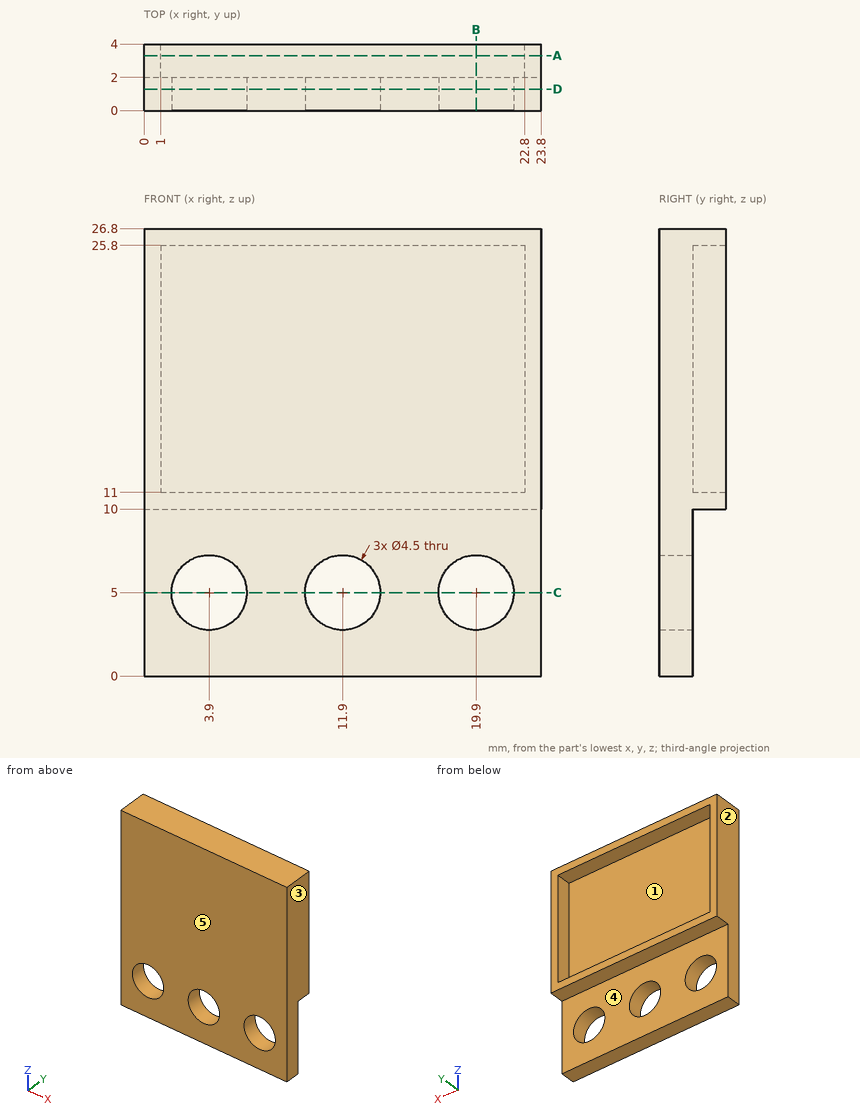
Job drawing, mm, ordinate dimensions from the low corner. One solid piece. A direction names the side the tool comes from. Coordinates: 2 decimals unless noted, no trailing zeros. Write each loop counter-clockwise with the first axis right and the second up, starting at its lowest first coordinate (ties: lowest second). Pieces come first, ordered by that corner, then holes.
Item 1: Slice it at A-A (y = 3.3). Write the cut outline in (x, z).
Item 2: Slice it at C-C (z = 5). Write the cut outline in (x, y).
Item 3: Pin check, flat tips, straight feed: pin 1 (6 mm diameter, centred on x = 19.9, z = 5, fed in from +Y); pin 2 (0.6 mm diameter, centred on x = 15.5, y = 2.5, fed in from -Z). Stop position of each tip, or through.
Item 4: Probe line 1 (X direction, y = 0.9, z = 5); line 2 (X direction, y = 2.7, z = 25.5); line 3 (Z direction, x = 7.25, y = 3.6). List the from-to ranges inside material, lowest first.
Item 5: Slice it at D-D (y = 1.3). Write the cut outline in (x, z), and give its area (3 significant figures).
Item 6: Which spindle directions (+Z, -Z, +X, -X, +Y, -Y) get a long thin tool onto all of the face, cutting with end or side? Do the marked faces 4 and 5. Say none if no direction does.
Item 7: Slice it at B-B (x = 19.9). Write the cut outline in (y, z), and give its area (3 significant figures).
Item 8: Mould opens along X. For the marked faces 1, 2 and 3 say: released by +X, released by -X, zero draft, split by the parting line, or undercut.
Results found:
1. outline: (0, 10) - (23.8, 10) - (23.8, 26.8) - (0, 26.8) - close; hole (1, 11) - (22.8, 11) - (22.8, 25.8) - (1, 25.8) - close
2. outline: (0, 0) - (1.65, 0) - (1.65, 2) - (0, 2) - close; (6.15, 0) - (9.65, 0) - (9.65, 2) - (6.15, 2) - close; (14.15, 0) - (17.65, 0) - (17.65, 2) - (14.15, 2) - close; (22.15, 0) - (23.8, 0) - (23.8, 2) - (22.15, 2) - close
3. pin 1: stops at y = 2
3. pin 2: stops at z = 10
4. line 1: x = 0 to 1.65, 6.15 to 9.65, 14.15 to 17.65, 22.15 to 23.8
4. line 2: x = 0 to 1, 22.8 to 23.8
4. line 3: z = 10 to 11, 25.8 to 26.8
5. outline: (0, 0) - (23.8, 0) - (23.8, 26.8) - (0, 26.8) - close; hole circle Ø4.5 at (3.9, 5); hole circle Ø4.5 at (11.9, 5); hole circle Ø4.5 at (19.9, 5)
5. area: 590 mm2
6. face 4: -Z, +X, -X, +Y
6. face 5: +Z, -Z, +X, -X, -Y
7. outline: (0, 0) - (2, 0) - (2, 2.75) - (0, 2.75) - close; (0, 7.25) - (2, 7.25) - (2, 10) - (4, 10) - (4, 11) - (2, 11) - (2, 25.8) - (4, 25.8) - (4, 26.8) - (0, 26.8) - close
7. area: 48.6 mm2
8. face 1: undercut
8. face 2: released by -X
8. face 3: released by +X
